The listing builds one solid part. Answer for the finished solid, in the listing's coordinates (mm). A direction names the side the tool comes from. Round coordinates to 2 decimals unless told otherwise and drop trailing zeros. Write each loop counter-clockwise with the first axis right and the second up, starting at its lowest first coordinate (ties: lowest second). Pieces come first, ordered by that corner, then holes.
from build123d import *

# Parameters (mm, degrees)
SKETCH1_W           = 178
SKETCH1_H           = 120
SKETCH1_R           = 11
SKETCH1_R_2         = 7.15
SKETCH1_W_2         = 138.4
SKETCH1_H_2         = 9.9
BOSS_EXTRUDE1_DEPTH = 9.5
M4_TAPPED_HOLE1_D   = 3.3


with BuildPart() as part:
    # Sketch1 → Boss-Extrude1 (new body)
    with BuildSketch(Plane(origin=(0, 0, 0), x_dir=(1, 0, 0), z_dir=(0, 1, 0))):
        Rectangle(SKETCH1_W, SKETCH1_H)
        with Locations((0, -28)):
            Circle(SKETCH1_R, mode=Mode.SUBTRACT)
        with Locations((-59, -24)):
            Circle(SKETCH1_R_2, mode=Mode.SUBTRACT)
        with Locations((59, -24)):
            Circle(SKETCH1_R_2, mode=Mode.SUBTRACT)
        with Locations((0, 44.95)):
            Rectangle(SKETCH1_W_2, SKETCH1_H_2, mode=Mode.SUBTRACT)
    extrude(amount=BOSS_EXTRUDE1_DEPTH)

    # M4 Tapped Hole1 (through all)
    with Locations(Plane(origin=(0, 9.5, 0), x_dir=(1, 0, 0), z_dir=(0, 1, 0))):
        with Locations((-80.25, 28), (0, 28), (80.25, 28)):
            Hole(M4_TAPPED_HOLE1_D / 2)


solid = part.part
1. Given pin 1 (2 mm diameter, centred on x = 80.25, z = -28, fed in from -Y) (3 decimals), flat-ended and moving along its own axis, determine where the tip first touches the part or whether it passes through.
Geometry says:
pin 1: passes through
2. A tool of negligible diameter and unlimited length cuts with its end or side. For faces 4 (the face through (-1, 5, -40)), 5 (the face through (89, 5, 1)), from which of +Z, -Z, +X, -X, +Y, -Y can it reach the whole face along a straight path? Write none if from no direction.
Geometry says:
face 4: +Y, -Y
face 5: +Z, -Z, +X, +Y, -Y
3. Section D-D on z = 28 is taken. Determine the outline of the cut face in (x, y).
Geometry says:
outline: (-89, 0) - (-64.93, 0) - (-64.93, 9.5) - (-89, 9.5) - close; (-53.07, 0) - (-11, 0) - (-11, 9.5) - (-53.07, 9.5) - close; (11, 0) - (53.07, 0) - (53.07, 9.5) - (11, 9.5) - close; (64.93, 0) - (89, 0) - (89, 9.5) - (64.93, 9.5) - close
4. Section A-A on x = -59 is taken. Determine the outline of the cut face in (y, z), plus the area to 3 significant figures.
Geometry says:
outline: (0, -60) - (9.5, -60) - (9.5, -49.9) - (0, -49.9) - close; (0, -40) - (9.5, -40) - (9.5, 16.85) - (0, 16.85) - close; (0, 31.15) - (9.5, 31.15) - (9.5, 60) - (0, 60) - close
area: 910 mm2
5. Section B-B on y = 5.25 is taken. Determine the outline of the cut face in (x, z), plus the area to 3 significant figures.
Geometry says:
outline: (-89, -60) - (89, -60) - (89, 60) - (-89, 60) - close; hole circle Ø3.3 at (-80.25, -28); hole (-69.2, -49.9) - (69.2, -49.9) - (69.2, -40) - (-69.2, -40) - close; hole circle Ø14.3 at (-59, 24); hole circle Ø22 at (0, 28); hole circle Ø3.3 at (0, -28); hole circle Ø14.3 at (59, 24); hole circle Ø3.3 at (80.25, -28)
area: 19,300 mm2
6. Section C-C on x = -33.5 is taken. Determine the outline of the cut face in (y, z).
Geometry says:
outline: (0, -60) - (9.5, -60) - (9.5, -49.9) - (0, -49.9) - close; (0, -40) - (9.5, -40) - (9.5, 60) - (0, 60) - close
7. Straight lines are drawn through the part: line 1 along Z through (x, y) = (0, 3.25); line 2 along Z through (x, y) = (-59, 5.5); line 3 along X through (y, z) = (2.5, -28). For each, find the intervals that lie inside material, in ascending order.
Geometry says:
line 1: z = -60 to -49.9, -40 to -29.65, -26.35 to 17, 39 to 60
line 2: z = -60 to -49.9, -40 to 16.85, 31.15 to 60
line 3: x = -89 to -81.9, -78.6 to -1.65, 1.65 to 78.6, 81.9 to 89
8. For a pull along Z with two mould halves and no side action, classify faces 1 (the face through (81.466, 4.684, -29.115)), 2 (the face through (-1, 9.5, -1)), 3 (the face through (-1, 5, -60)) as released by +Z, released by -Z, zero draft, split by the parting line, or undercut.
Geometry says:
face 1: undercut
face 2: zero draft
face 3: released by -Z
